Build history of the part. All positions in model axes, mm. A direction names the side the tool comes from. Give positions to 0.01 mm unless a question says otherwise; leave off trailing zeros. Write each loop counter-clockwise with the first axis right and the second up, starting at its lowest first coordinate (ties: lowest second). Pieces come first, ordered by that corner, then holes. Notation, with made-up numbers: (-19.5, 59) -> (-2.5, 59) arc R33 cw to (-2.5, 87) -> close; hole circle Ø7 at (-3.5, -39). An arc over 180 degrees is marked (long way). Put each result on its own line as item: value. Start each with the question number.
Item 1: Drill centre lines: line 1 along X through (y, z) = (-7.25, -12.25); line 2 along Z through (x, y) = (-10.5, -4); line 3 along Y through (x, z) = (-30, -7.5). Where is each one in solid material? Low to high.
Item 2: Slice it at C-C, the plane y = -5. List the corners of the cut face in (x, z).
Item 3: Slice it at D-D, the plane z = -2. List the corners of the cut face in (x, y).
Item 4: Slice it at B-B, the plane x = -23.5. List the corners of the cut face in (y, z), plus the area to 3 significant figures.
Item 5: Flat gauge pins, fed straight in: pin 1 Ø5 at (y, z) = (-10, -5.5) entering from +X; pin 2 Ø2 at (y, z) = (-0.5, -12) entering from +X; pin 3 Ø5 at (x, y) = (-6.5, -6) entering from -Z; pin 4 Ø2 at (y, z) = (-12.5, -4) entering from -X. Where does each tip first touch, or does it go through?
Item 6: Tool access for faces 1 (the flat face through (-2.5, -8, -7)), 2 (the flat face through (-29.5, -8, -7)), 3 (the flat face through (-16, -8, -2.5)), 4 (the flat face through (-16, -8, -12.5)): list every direction of +Z, -Z, +X, -X, +Y, -Y with a clear straight run to the whole face (end or side of a thin tool).
Item 7: Slice it at A-A, the plane z = -10. List the corners of the cut face in (x, y), plus the area to 3 significant figures.
```python
from build123d import *

# Parameters (mm, degrees)
SKETCH1_W           = 32
SKETCH1_H           = 15
BOSS_EXTRUDE1_DEPTH = 1.5
FILLET2_R           = 0.2
SKETCH2_W           = 27
SKETCH2_H           = 10
BOSS_EXTRUDE2_DEPTH = 18.5


with BuildPart() as part:
    # Sketch1 → Boss-Extrude1 (new body)
    with BuildSketch(Plane(origin=(0, 0, 0), x_dir=(1, 0, 0), z_dir=(0, 1, 0))):
        with Locations((-16, 7.5)):
            Rectangle(SKETCH1_W, SKETCH1_H)
    extrude(amount=BOSS_EXTRUDE1_DEPTH)

    # Fillet2
    fillet2_edges = [part.edges().sort_by_distance(p)[0] for p in [
        (-32, 1.5, -7.5),
        (-16, 1.5, 0),
        (0, 1.5, -7.5),
        (-16, 1.5, -15),
        (0, 0.75, 0),
        (-32, 0.75, 0),
        (-32, 0.75, -15),
        (0, 0.75, -15),
    ]]
    fillet(fillet2_edges, radius=FILLET2_R)

    # Sketch2 → Boss-Extrude2 (add)
    with BuildSketch(Plane(origin=(0, 1.5, 0), x_dir=(1, 0, 0), z_dir=(0, 1, 0))):
        with Locations((-16, 7.5)):
            Rectangle(SKETCH2_W, SKETCH2_H)
    extrude(amount=-BOSS_EXTRUDE2_DEPTH)


solid = part.part
```
Values follow:
1. line 1: -29.5 to -2.5
1. line 2: -12.5 to -2.5
1. line 3: 0 to 1.5
2. outline: (-29.5, -12.5) -> (-2.5, -12.5) -> (-2.5, -2.5) -> (-29.5, -2.5) -> close
3. outline: (-32, 0) -> (0, 0) -> (0, 1.3) arc R0.2 ccw to (-0.2, 1.5) -> (-31.8, 1.5) arc R0.2 ccw to (-32, 1.3) -> close
4. outline: (-17, -12.5) -> (0, -12.5) -> (0, -15) -> (1.3, -15) arc R0.2 ccw to (1.5, -14.8) -> (1.5, -0.2) arc R0.2 ccw to (1.3, 0) -> (0, 0) -> (0, -2.5) -> (-17, -2.5) -> close
4. area: 192 mm2
5. pin 1: x = -2.5
5. pin 2: x = 0
5. pin 3: z = -12.5
5. pin 4: x = -29.5
6. face 1: +Z, -Z, +X, -Y
6. face 2: +Z, -Z, -X, -Y
6. face 3: +Z, +X, -X, -Y
6. face 4: -Z, +X, -X, -Y
7. outline: (-32, 0) -> (-29.5, 0) -> (-29.5, -17) -> (-2.5, -17) -> (-2.5, 0) -> (0, 0) -> (0, 1.3) arc R0.2 ccw to (-0.2, 1.5) -> (-31.8, 1.5) arc R0.2 ccw to (-32, 1.3) -> close
7. area: 507 mm2
